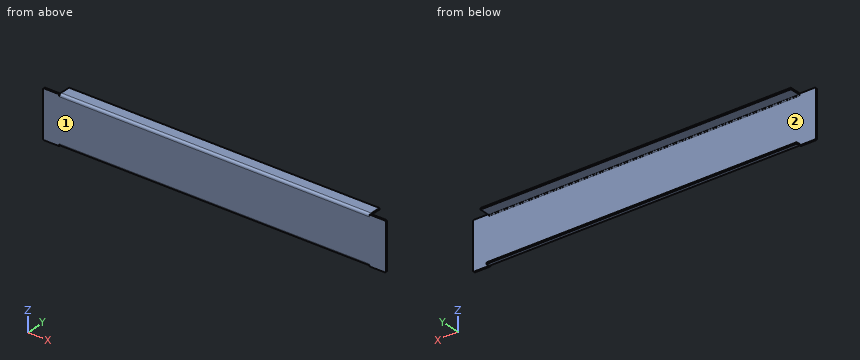
from build123d import *

# Parameters (mm, degrees)
FLANGE_BASE2_DEPTH       = 137.5
CORTE_EXTRUS_O3_START    = -137.5
CORTE_EXTRUS_O3_DEPTH    = 13
CORTE_EXTRUS_O3_START_2  = 124.5
CORTE_EXTRUS_O3_2_DEPTH  = 13
ESBO_O12_W               = 13
ESBO_O12_H               = 1.2
RESSALTO_EXTRUS_O1_DEPTH = 19
FILETE1_R                = 1


# Read off the part's stored shape, not the designer's step: Corte-extrusão3
# Sheet-metal steps are written as plain solids
with BuildPart() as part:
    # Esboço1 → Flange-base2 (new, symmetric)
    with BuildSketch(Plane(origin=(0, 0, 0), x_dir=(0, 0, -1), z_dir=(1, 0, 0))):
        with BuildLine():
            Line((-18, 9), (-18, 0.7366))
            ThreePointArc((-18, 0.7366), (-17.784254855, 0.215745145), (-17.2634, 0))
            Line((-17.2634, 0), (17.2634, 0))
            ThreePointArc((17.2634, 0), (17.784254855, 0.215745145), (18, 0.7366))
            Line((18, 0.7366), (18, 3))
            Line((18, 3), (19.2, 3))
            Line((19.2, 3), (19.2, 0.7366))
            ThreePointArc((19.2, 0.7366), (18.632782992, -0.632782992), (17.2634, -1.2))
            Line((17.2634, -1.2), (-17.2634, -1.2))
            ThreePointArc((-17.2634, -1.2), (-18.632782992, -0.632782992), (-19.2, 0.7366))
            Line((-19.2, 0.7366), (-19.2, 9))
            Line((-19.2, 9), (-18, 9))
        make_face()
    extrude(amount=FLANGE_BASE2_DEPTH, both=True)

    # Corte-extrusão3 outline → Corte-extrusão3 (cut)
    with BuildSketch(Plane.YZ.offset(CORTE_EXTRUS_O3_START)):
        with BuildLine():
            Line((-1.2, 17.2634), (0, 17.2634))
            ThreePointArc((0, 17.2634), (0.215745145, 17.784254855), (0.7366, 18))
            Line((0.7366, 18), (9, 18))
            Line((9, 18), (9, 19.2))
            Line((9, 19.2), (0.7366, 19.2))
            ThreePointArc((0.7366, 19.2), (-0.632782992, 18.632782992), (-1.2, 17.2634))
        make_face()
        with BuildLine():
            ThreePointArc((0.7366, -18), (0.215745145, -17.784254855), (0, -17.2634))
            Line((0, -17.2634), (-1.2, -17.2634))
            ThreePointArc((-1.2, -17.2634), (-0.632782992, -18.632782992), (0.7366, -19.2))
            Line((0.7366, -19.2), (3, -19.2))
            Line((3, -19.2), (3, -18))
            Line((3, -18), (0.7366, -18))
        make_face()
    extrude(amount=CORTE_EXTRUS_O3_DEPTH, mode=Mode.SUBTRACT)

    # Corte-extrus_o3 2 outline → Corte-extrus_o3 2 (cut)
    with BuildSketch(Plane.YZ.offset(CORTE_EXTRUS_O3_START_2)):
        with BuildLine():
            Line((-1.2, 17.2634), (0, 17.2634))
            ThreePointArc((0, 17.2634), (0.215745145, 17.784254855), (0.7366, 18))
            Line((0.7366, 18), (9, 18))
            Line((9, 18), (9, 19.2))
            Line((9, 19.2), (0.7366, 19.2))
            ThreePointArc((0.7366, 19.2), (-0.632782992, 18.632782992), (-1.2, 17.2634))
        make_face()
        with BuildLine():
            ThreePointArc((0.7366, -18), (0.215745145, -17.784254855), (0, -17.2634))
            Line((0, -17.2634), (-1.2, -17.2634))
            ThreePointArc((-1.2, -17.2634), (-0.632782992, -18.632782992), (0.7366, -19.2))
            Line((0.7366, -19.2), (3, -19.2))
            Line((3, -19.2), (3, -18))
            Line((3, -18), (0.7366, -18))
        make_face()
    extrude(amount=CORTE_EXTRUS_O3_2_DEPTH, mode=Mode.SUBTRACT)

    # Esboço12 → Ressalto-extrusão1 (add, symmetric)
    with BuildSketch(Plane.XY):
        with Locations((131, -0.6)):
            Rectangle(ESBO_O12_W, ESBO_O12_H)
        with Locations((-131, -0.6)):
            Rectangle(ESBO_O12_W, ESBO_O12_H)
    extrude(amount=RESSALTO_EXTRUS_O1_DEPTH, both=True)

    # Filete1
    filete1_edges = [part.edges().sort_by_distance(p)[0] for p in [
        (137.5, -0.6, -19),
        (137.5, -0.6, 19),
        (-137.5, -0.6, -19),
        (-137.5, -0.6, 19),
    ]]
    fillet(filete1_edges, radius=FILETE1_R)


solid = part.part
For this review, take the finished solid that the model builds, in its own axes (mm). Face numbers are marked on the shaded views. Coordinates: 2 decimals unless noted, no trailing zeros. Loops run counter-clockwise (first coordinate to the right, second up) from the corner with the lowest first, then second, coordinate; pieces in that order, holes last. Notation, with made-up numbers: (68.5, 9.25) - (108.5, 9.25) arc R38 ccw to (108.5, 47.25) - close; hole circle Ø7 at (89.25, 31). An arc over 180 degrees is marked (long way). Use a Markdown table: item, result. Add a question column.
Item 1: Mouldability with a two-part tool opening along Z and no side actions: class the marked faces 1 and 2 as pulls with the +Z half, pulls with the -Z half, needs draft (parallel to the pull), parting line crosses it, or undercut.
Item 2: We need section B-B (z = 10). Give the boundary of the cut face in (x, y).
Item 3: We need section A-A (x = 20). Give the boundary of the cut face in (y, z).
Item 4: We need section C-C (y = 5). Give the boundary of the cut face in (x, z).
Item 5: Insertion check: pin 1 Ø0.6 at (x, y) = (-133.5, -0.5) entering from -Z; pin 2 Ø0.5 at (y, z) = (-1, -18.5) entering from +X; pin 3 Ø1.5 at (x, z) = (-88.5, 11.5) entering from +Y; pin 4 Ø1 at (y, z) = (2, 0.5) entering from +X. Each pin has a flat end and moves straight along its axis. Give the tip position at first contact, or say it passes through.
Item 6: For line 1 (Z direction, x = -12.5, y = 2); line 2 (Y direction, x = -8.5, z = 13); line 3 (Z direction, x = 120.5, y = 7.75), list the stretches that pass through material, from the lowest coordinate up.
Results list:
| question | item | result |
|---|---|---|
| 1 | face 1 | needs draft |
| 1 | face 2 | undercut |
| 2 | outline | (-137.5, -1.2) - (137.5, -1.2) - (137.5, 0) - (-137.5, 0) - close |
| 3 | outline | (-1.2, -17.26) arc R1.94 ccw to (0.74, -19.2) - (3, -19.2) - (3, -18) - (0.74, -18) arc R0.74 cw to (0, -17.26) - (0, 17.26) arc R0.74 cw to (0.74, 18) - (9, 18) - (9, 19.2) - (0.74, 19.2) arc R1.94 ccw to (-1.2, 17.26) - close |
| 4 | outline | (-124.5, 18) - (124.5, 18) - (124.5, 19.2) - (-124.5, 19.2) - close |
| 5 | pin 1 | stops at z = -19 |
| 5 | pin 2 | stops at x = 137.47 |
| 5 | pin 3 | stops at y = 0 |
| 5 | pin 4 | passes through |
| 6 | line 1 | z = -19.2 to -18, 18 to 19.2 |
| 6 | line 2 | y = -1.2 to 0 |
| 6 | line 3 | z = 18 to 19.2 |
